from build123d import *

# Parameters (mm, degrees)
F0_R     = 15
F0_R_2   = 3.05
F0_R_3   = 3
F1_DEPTH = 20
F2_DEPTH = 1
F3_R     = 15
F4_DEPTH = 1.5
F6_START = 5
F5_R     = 1
F5_R_2   = 1.5
F6_DEPTH = 20
F8_DEPTH = 25
F9_SIZE  = 0.5


with BuildPart() as f1:
    # F0 (on Top) → F1 (new body)
    with BuildSketch(Plane.XY):
        Circle(F0_R)
        with Locations((-7.05, 0)):
            Circle(F0_R_2, mode=Mode.SUBTRACT)
        Circle(F0_R_3, mode=Mode.SUBTRACT)
        with Locations((7.05, 0)):
            Circle(F0_R_2, mode=Mode.SUBTRACT)
    extrude(amount=F1_DEPTH)

    # F0 (on Top) → F2 (join)
    with BuildSketch(Plane.XY):
        with Locations((-7.05, 0)):
            Circle(F0_R_2)
        with Locations((7.05, 0)):
            Circle(F0_R_2)
    extrude(amount=F2_DEPTH)

    # F3 (on face) → F4 (cut)
    with BuildSketch(Plane.XY.offset(20)):
        Circle(F3_R)
        with BuildLine():
            ThreePointArc((-6.8546099291, 3.0437349951), (0, 7.5), (6.8546099291, 3.0437349951))
            ThreePointArc((6.8546099291, 3.0437349951), (9.1364515671, 2.2246842154), (10.1, 0))
            ThreePointArc((10.1, 0), (9.1364515671, -2.2246842154), (6.8546099291, -3.0437349951))
            ThreePointArc((6.8546099291, -3.0437349951), (0, -7.5), (-6.8546099291, -3.0437349951))
            ThreePointArc((-6.8546099291, -3.0437349951), (-10.1, 0), (-6.8546099291, 3.0437349951))
        make_face(mode=Mode.SUBTRACT)
    extrude(amount=-F4_DEPTH, mode=Mode.SUBTRACT)

    # F5 (on Front) → F6 (cut)
    with BuildSketch(Plane.XZ.offset(F6_START)):
        with Locations((0, 4.5)):
            Circle(F5_R)
        with Locations((0, 8)):
            Circle(F5_R_2)
    extrude(amount=F6_DEPTH, mode=Mode.SUBTRACT)

    # F7 (on face) → F8 (cut)
    with BuildSketch(Plane.XY):
        with BuildLine():
            Line((6.5383484153, -13.5), (-6.5383484153, -13.5))
            ThreePointArc((-6.5383484153, -13.5), (0, -15), (6.5383484153, -13.5))
        make_face()
    extrude(amount=F8_DEPTH, mode=Mode.SUBTRACT)

    # F9
    f9_edges = [f1.edges().sort_by_distance(p)[0] for p in [
        (0, 15, 0),
        (0, -13.5, 0),
        (-3, 0, 0),
        (0, 15, 18.5),
        (-3, 0, 20),
        (0, -13.5, 18.5),
    ]]
    chamfer(f9_edges, length=F9_SIZE)


solid = f1.part
Geometry: final body of the model. Coordinates: model frame, mm. A direction names the side the tool comes from. Give positions to 0.01 mm unless a question says otherwise; leave off trailing zeros. Write each loop counter-clockwise with the first axis right and the second up, starting at its lowest first coordinate (ties: lowest second). Pieces come first, ordered by that corner, then holes. Notation, with made-up numbers: M 36,-28 L 78,-28 A17 cw 78,-22 Z; hole C -15,61.25 d8. An arc over 180 degrees is marked long. Answer in a Markdown table with one row per item. Add a question column.
(1) Section A-A on y = 0. Return loops of the section in (x, z), and give its area (4 significant figures).
(2) Reachability of faces 1 (the flat face through (-1.6, 3.4, 20)), 2 (the cylindrical face through (0.1, -7.5, 19.3)), 3 (the cylindrical face through (-0.13, -9.19, 5.49)), 4 (the flat face through (7, 0, 1)) from +Z, -Z, +X, -X, +Y, -Y: full face, straight path, thin tool, end or side. Return the list, or none.
(3) Section C-C on x = 0. Return loops of the section in (y, z).
(4) Section B-B on z = 4.5. Return loops of the section in (x, y).
(5) Mould query, pull axis Z, two halves, no side actions, for faces 5 (the conical face through (-0.55, 14.63, 0.14)), 6 (the flat face through (0, -5, 8)), 7 (the cylindrical face through (-0.1, 7.5, 19.3)), 8 (the flat face through (0, -5, 5)). Classes: +Z half, -Z half, draft (parallel to the pull), parting line (faces both ways), or undercut.
(6) Section D-D on z = 8. Return loops of the section in (x, y).
(7) First-contact query: pin 1 (8 mm diameter, centred on y = -8, z = 3.5, fed in from -X); pin 2 (1 mm diameter, centred on x = 0, z = 4.5, fed in from -Y); pin 3 (10 mm diameter, centred on y = 7, z = 15, fed in from +X). Flat tips, straight axial feed; report the tip coordinate or a pass-through.
(8) Ray query, line 1 (Z direction, x = 0, y = -7); line 2 (Z direction, x = 0, y = -10); line 3 (Y direction, x = 0, z = 5.75). Return the intervals inside material, ascending.
Result set:
| question | item | result |
|---|---|---|
| 1 | outline | M -15,0.5 L -14.5,0 L -3.5,0 L -3,0.5 L -3,19.5 L -3.5,20 L -4,20 L -4,1 L -10.1,1 L -10.1,18.5 L -14.5,18.5 L -15,18 Z; M 3,0.5 L 3.5,0 L 14.5,0 L 15,0.5 L 15,18 L 14.5,18.5 L 10.1,18.5 L 10.1,1 L 4,1 L 4,20 L 3.5,20 L 3,19.5 Z |
| 1 | area | 232.5 mm^2 |
| 2 | face 1 | +Z, +X, -X, +Y, -Y |
| 2 | face 2 | +Z, -Y |
| 2 | face 3 | -Y |
| 2 | face 4 | +Z |
| 3 | outline | M -13.5,0.5 L -13,0 L -3.5,0 L -3,0.5 L -3,19.5 L -3.5,20 L -7.5,20 L -7.5,18.5 L -13,18.5 L -13.5,18 L -13.5,9.5 L -5,9.5 L -5,6.5 L -13.5,6.5 L -13.5,5.5 L -5,5.5 L -5,3.5 L -13.5,3.5 Z; M 3,0.5 L 3.5,0 L 14.5,0 L 15,0.5 L 15,18 L 14.5,18.5 L 7.5,18.5 L 7.5,20 L 3.5,20 L 3,19.5 Z |
| 4 | outline | M -6.54,-13.5 L -1,-13.5 L -1,-5 L 1,-5 L 1,-13.5 L 6.54,-13.5 A15 ccw long Z; hole C -7.05,0 d6.1; hole C 0,0 d6; hole C 7.05,0 d6.1 |
| 5 | face 5 | -Z half |
| 5 | face 6 | undercut |
| 5 | face 7 | draft |
| 5 | face 8 | undercut |
| 6 | outline | M -6.54,-13.5 L -1.5,-13.5 L -1.5,-5 L 1.5,-5 L 1.5,-13.5 L 6.54,-13.5 A15 ccw long Z; hole C -7.05,0 d6.1; hole C 0,0 d6; hole C 7.05,0 d6.1 |
| 7 | pin 1 | stops at x = -14.46 |
| 7 | pin 2 | stops at y = -5 |
| 7 | pin 3 | stops at x = 14.87 |
| 8 | line 1 | z = 0 to 3.5, 5.5 to 6.5, 9.5 to 20 |
| 8 | line 2 | z = 0 to 3.5, 5.5 to 6.5, 9.5 to 18.5 |
| 8 | line 3 | y = -13.5 to -3, 3 to 15 |
